```python
from build123d import *

# Parameters (mm, degrees)
BOSS_EXTRUDE2_REACH      = 18.583
BOSS_EXTRUDE2_END_RADIUS = 5
SKETCH2_R                = 2
FILLET1_R                = 2


with BuildPart() as part:
    # Sketch1 → Revolve1 (revolve)
    with BuildSketch(Plane.XY):
        with BuildLine():
            Line((0, 5), (0, -5))
            ThreePointArc((0, -5), (-5, 0), (0, 5))
        make_face()
    revolve(axis=Axis((0, 5, 0), (0, -1, 0)))

    # Boss-Extrude2: up to this sphere (the profile starts outside it)
    boss_extrude2_end = Location((0, 0, 0)) * Sphere(BOSS_EXTRUDE2_END_RADIUS, mode=Mode.PRIVATE)
    # Sketch2 → Boss-Extrude2 (add, up to the surface)
    with BuildSketch(Plane(origin=(0, 10, 0), x_dir=(1, 0, 0), z_dir=(0, 1, 0)), mode=Mode.PRIVATE) as boss_extrude2_sk1:
        with Locations(Location((0, 0, 0), (0, 0, 270))):
            Circle(SKETCH2_R)
    boss_extrude2_tool1 = extrude(boss_extrude2_sk1.sketch, amount=-BOSS_EXTRUDE2_REACH, mode=Mode.PRIVATE) - boss_extrude2_end
    add(boss_extrude2_tool1.solids().sort_by_distance((0, 10, 0))[0])

    # Fillet1
    fillet1_edges = [part.edges().sort_by_distance(p)[0] for p in [
        (1.414213562, 4.582575695, -1.414213562),
    ]]
    fillet(fillet1_edges, radius=FILLET1_R)


solid = part.part
```
For this review, take the finished solid that the model builds, in its own axes (mm). A direction names the side the tool comes from. Coordinates: 2 decimals unless noted, no trailing zeros. Loops run counter-clockwise (first coordinate to the right, second up) from the corner with the lowest first, then second, coordinate; pieces in that order, holes last. Notation, with made-up numbers: (86.25, -17.5) - (134.25, -17.5) arc R9 cw to (134.25, -2.5) - close; hole circle Ø3 at (-25, -23.75). An arc over 180 degrees is marked (long way). Use one line per item in the form item = value. Start each with the question number.
1) Take a section at A-A (y = -3). State the section outline as (x, z) points, plus the area to 3 significant figures.
2) To check wall thickness, follow probe 1 along X at (y, z) = (-3, 1.5); probe 2 along Z at (x, y) = (-1.25, -1.5); probe 3 along Y at (x, z) = (-0.75, 1.5). State the ranges of each line that lie inside material, in increasing order. Write a range as from..to.
3) For faces 1 (the face through (-2, 8, 0)), 2 (the face through (0, 10, 0)), list the 3-axis set-ups (+Z, -Z, +X, -X, +Y, -Y) from which the entire face can be reached by the end or side of a thin tool; tool diameter is ignored.
4) For pin 1 (4 mm diameter, centred on y = 6.5, z = -1, fed in from +X); pin 2 (1 mm diameter, centred on x = -0.5, z = 2, fed in from -Y); pin 3 (3 mm diameter, centred on x = -3, y = 5, fed in from +Z); pin 4 (2 mm diameter, centred on y = 7, z = -3.5, fed in from -X), all flat-tipped, find the tip position at first contact; note any pin that passes through.
5) Take a section at B-B (x = -3.25). State the section outline as (y, z) points.
From the geometry:
q1.outline = circle Ø8 at (0, 0)
q1.area = 50.3 mm2
q2.probe_1 = -3.71..3.71
q2.probe_2 = -4.6..4.6
q2.probe_3 = -4.71..10
q3.face_1 = +Y
q3.face_2 = +Z, -Z, +X, -X, +Y
q4.pin_1 = 2.33
q4.pin_2 = -4.75
q4.pin_3 = 2.5
q4.pin_4 = through
q5.outline = circle Ø7.6 at (0, 0)
